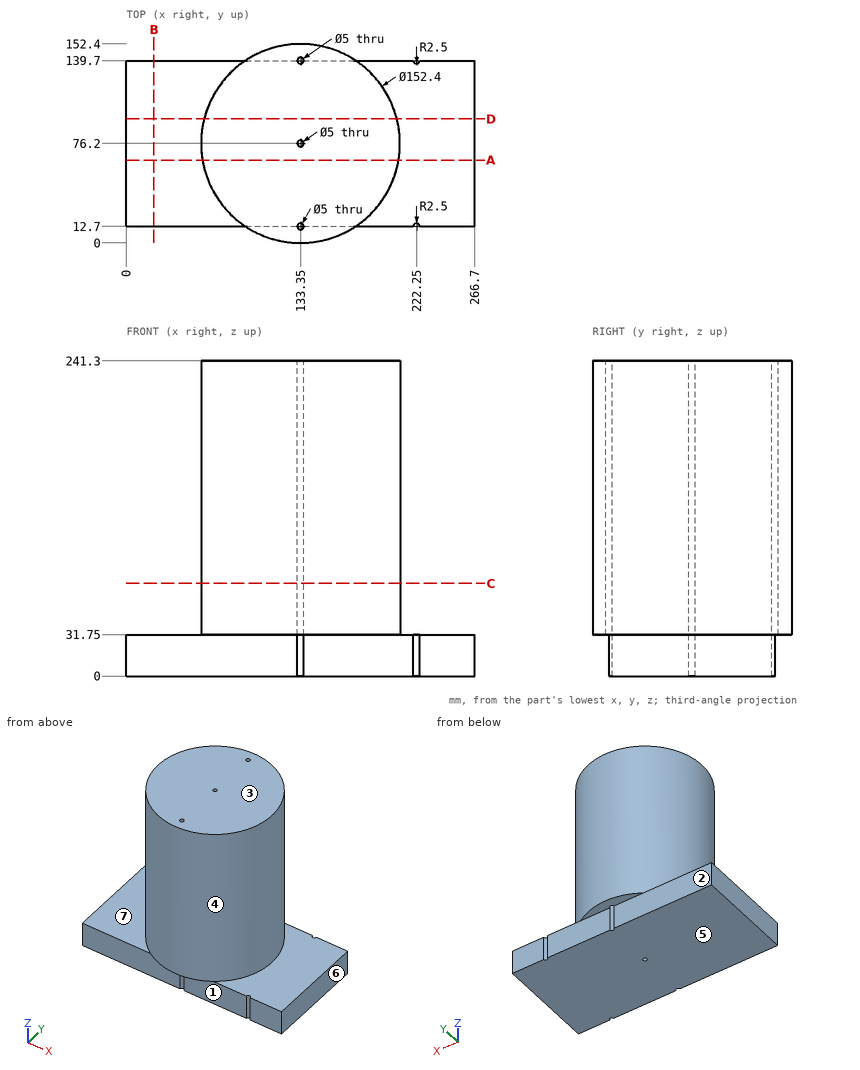
Study the drawing (mm; zero at the part's minimum x, y, z) and answer. A direction names the side the tool comes from. Give positions to 0.01 mm unless a question says otherwise; leave off trailing zeros. Order: outer loops, then holes, each group sorted by start corner. A loop starts at its lowest first (then second) coordinate and runs counter-clockwise, first axis right, second up. Notation, with made-up numbers: (16, 40) -> (52, 40) arc R38 ccw to (52, 78) -> close; hole circle Ø10 at (54, 70). An arc over 180 degrees is marked (long way). Put each result on its own line as item: value.
Item 1: A cutting plane is placed at D-D on y = 95. Give the vertices of the cut face in (x, z), plus the area to 3 significant figures.
Established:
outline: (0, 0) -> (266.7, 0) -> (266.7, 31.75) -> (207.19, 31.75) -> (207.19, 241.3) -> (59.51, 241.3) -> (59.51, 31.75) -> (0, 31.75) -> close
area: 39,400 mm^2
Item 2: For the marked faces 1, 2, 3 and 4, determine the directions among +Z, -Z, +X, -X, +Y, -Y from which every point of the face is accessible in a straight line to the end or side of a thin tool.
Established:
face 1: -Z, +X, -X, -Y
face 2: -Z, +X, -X, +Y
face 3: +Z, +X, -X, +Y, -Y
face 4: +Z
Item 3: A cutting plane is placed at A-A on y = 63.5. Give the vertices of the cut face in (x, z).
Established:
outline: (0, 0) -> (266.7, 0) -> (266.7, 31.75) -> (208.48, 31.75) -> (208.48, 241.3) -> (58.22, 241.3) -> (58.22, 31.75) -> (0, 31.75) -> close
Item 4: A cutting plane is placed at C-C on z = 71. Give the vertices of the cut face in (x, y).
Established:
outline: circle Ø152.4 at (133.35, 76.2); hole circle Ø5 at (133.35, 12.7); hole circle Ø5 at (133.35, 76.2); hole circle Ø5 at (133.35, 139.7)
Item 5: A cutting plane is placed at B-B on x = 21. Give the vertices of the cut face in (y, z).
Established:
outline: (12.7, 0) -> (139.7, 0) -> (139.7, 31.75) -> (12.7, 31.75) -> close
Item 6: Straight lines are drawn through the part: line 1 (Y direction, x = 133, z = 85); line 2 (X direction, y = 76.2, z = 138); line 3 (X direction, y = 12.7, z = 179). For each, find the intervals that lie inside material, in ascending order.
Established:
line 1: y = 0 to 10.22, 15.18 to 73.72, 78.68 to 137.22, 142.18 to 152.4
line 2: x = 57.15 to 130.85, 135.85 to 209.55
line 3: x = 91.23 to 130.85, 135.85 to 175.47
Item 7: Given P1, Ø10, axis at x = 163, z = 48, coming from the +Y side; P2, Ø1.5, axis at y = 137, z = 159, coming from the +X side; P3, Ø9.5, axis at x = 188, z = 8.5, coming from the -Y side, each flat-ended and moving along its own axis, determine where each tip first touches the part or whether it passes through.
Established:
P1: stops at y = 148.3
P2: stops at x = 180.26
P3: stops at y = 12.7
Item 8: For a pull along Z with two mould halves and no side action, classify the marked faces 5, 6 and 7 as released by +Z, released by -Z, zero draft, split by the parting line, or undercut.
Established:
face 5: released by -Z
face 6: zero draft
face 7: released by +Z
